from build123d import *

# Parameters (mm, degrees)
SKETCH1_W           = 31.86
SKETCH1_H           = 328
BOSS_EXTRUDE1_DEPTH = 5
SKETCH2_R           = 2.1
CUT_EXTRUDE1_DEPTH  = 10
CUT_EXTRUDE2_DEPTH  = 10
BOSS_EXTRUDE2_DEPTH = 5
SKETCH7_W           = 4.2
SKETCH7_H           = 5
SKETCH7_R           = 2.099999245
CUT_EXTRUDE3_DEPTH  = 5
SKETCH8_R           = 2.499996422
SKETCH8_R_2         = 2.499996502
SKETCH8_R_3         = 2.5
SKETCH8_W           = 40.200355047
SKETCH8_H           = 20
CUT_EXTRUDE4_DEPTH  = 10
CUT_EXTRUDE5_DEPTH  = 10
CUT_EXTRUDE6_DEPTH  = 10
SKETCH12_R          = 2.100000755
SKETCH12_R_2        = 2.1
SKETCH12_W          = 15.000005391
SKETCH12_H          = 5
SKETCH12_W_2        = 5
SKETCH12_H_2        = 40
CUT_EXTRUDE7_DEPTH  = 5
SKETCH15_W          = 40
SKETCH15_H          = 5
CUT_EXTRUDE8_DEPTH  = 5


with BuildPart() as part:
    # Sketch1 → Boss-Extrude1 (new body)
    with BuildSketch(Plane.XY):
        Rectangle(SKETCH1_W, SKETCH1_H)
    extrude(amount=BOSS_EXTRUDE1_DEPTH)

    # Sketch2 → Cut-Extrude1 (cut)
    with BuildSketch(Plane.XY.offset(5)):
        with Locations((0, 81.5)):
            Circle(SKETCH2_R)
    extrude(amount=-CUT_EXTRUDE1_DEPTH, mode=Mode.SUBTRACT)

    # Sketch3 → Cut-Extrude2 (cut)
    with BuildSketch(Plane.XY.offset(5)):
        Polygon((2.1, 164), (2.1, 159), (5, 159), (5, 149), (-5, 149), (-5, 159), (-2.1, 159), (-2.1, 164), align=None)
        Polygon((-2.1, -164), (-2.1, -159), (-5, -159), (-5, -149), (5, -149), (5, -159), (2.1, -159), (2.1, -164), align=None)
    extrude(amount=-CUT_EXTRUDE2_DEPTH, mode=Mode.SUBTRACT)

    # Sketch4 → Boss-Extrude2 (add)
    with BuildSketch(Plane(origin=(0, 0, 0), x_dir=(-1, 0, 0), z_dir=(0, 0, -1))):
        with BuildLine():
            Line((15.93, -164), (108.913444487, -164))
            Line((108.913444487, -164), (108.913444487, 109))
            Line((108.913444487, 109), (101.503490547, 109))
            ThreePointArc((101.503490547, 109), (62.423444487, 88.5), (23.343398428, 109))
            ThreePointArc((23.343398428, 109), (18.773737927, 117.266257257), (15.93, 126.273252357))
            Line((15.93, 126.273252357), (15.93, 109))
            Line((15.93, 109), (15.93, -164))
        make_face()
    extrude(amount=-BOSS_EXTRUDE2_DEPTH)

    # Sketch7 → Cut-Extrude3 (cut)
    with BuildSketch(Plane.XY.offset(5)):
        Polygon((-95.083444487, -159), (-90.883444487, -159), (-87.983444487, -159), (-87.983444487, -149), (-97.983444487, -149), (-97.983444487, -159), align=None)
        with Locations((-92.983444487, -161.5)):
            Rectangle(SKETCH7_W, SKETCH7_H)
        with Locations((0.021526005, 106.5)):
            Circle(SKETCH7_R)
    extrude(amount=-CUT_EXTRUDE3_DEPTH, mode=Mode.SUBTRACT)

    # Sketch8 → Cut-Extrude4 (cut)
    with BuildSketch(Plane.XY.offset(5)):
        with Locations((-38.679067758, 44.08)):
            Circle(SKETCH8_R)
        with Locations((-38.679067758, 33.92)):
            Circle(SKETCH8_R_2)
        with Locations((10.13, 44.08)):
            Circle(SKETCH8_R_3)
        with Locations((10.13, 33.92)):
            Circle(SKETCH8_R_3)
        with Locations((-14.269822477, 39)):
            Rectangle(SKETCH8_W, SKETCH8_H)
    extrude(amount=-CUT_EXTRUDE4_DEPTH, mode=Mode.SUBTRACT)

    # Sketch9 → Cut-Extrude5 (cut)
    with BuildSketch(Plane(origin=(0, 0, 0), x_dir=(-1, 0, 0), z_dir=(0, 0, -1))):
        with BuildLine():
            Line((4.37, 12), (4.37, 19))
            ThreePointArc((4.37, 19), (-15.63, 39), (4.37, 59))
            Line((4.37, 59), (4.37, 66))
            ThreePointArc((4.37, 66), (-22.63, 39), (4.37, 12))
        make_face()
    extrude(amount=-CUT_EXTRUDE5_DEPTH, mode=Mode.SUBTRACT)

    # Sketch10 → Cut-Extrude6 (cut)
    with BuildSketch(Plane(origin=(0, 0, 0), x_dir=(-1, 0, 0), z_dir=(0, 0, -1))):
        with BuildLine():
            Line((-15.93, 66), (-15.93, 56.801966184))
            ThreePointArc((-15.93, 56.801966184), (-6.773314432, 63.593221495), (4.37, 66))
            Line((4.37, 66), (4.25, 81.5))
            ThreePointArc((4.25, 81.5), (0, 77.25), (-4.25, 81.5))
            Line((-4.25, 81.5), (-15.93, 81.5))
            Line((-15.93, 81.5), (-15.93, 66))
        make_face()
    extrude(amount=-CUT_EXTRUDE6_DEPTH, mode=Mode.SUBTRACT)

    # Sketch12 → Cut-Extrude7 (cut)
    with BuildSketch(Plane(origin=(0, 0, 0), x_dir=(-1, 0, 0), z_dir=(0, 0, -1))):
        with Locations((30.403186809, -93.5)):
            Circle(SKETCH12_R)
        with Locations((79.236368236, -70)):
            Circle(SKETCH12_R_2)
        with Locations((54.236365541, -93.5)):
            Rectangle(SKETCH12_W, SKETCH12_H)
        with Locations((6.570008077, -93.5)):
            Rectangle(SKETCH12_W, SKETCH12_H)
        with Locations((79.236368236, -114)):
            Rectangle(SKETCH12_W_2, SKETCH12_H_2)
        with Locations((79.236368236, -26)):
            Rectangle(SKETCH12_W_2, SKETCH12_H_2)
    extrude(amount=-CUT_EXTRUDE7_DEPTH, mode=Mode.SUBTRACT)

    # Sketch15 → Cut-Extrude8 (cut)
    with BuildSketch(Plane.XY.offset(5)):
        with Locations((-61.674975637, 81.5)):
            Rectangle(SKETCH15_W, SKETCH15_H)
    extrude(amount=-CUT_EXTRUDE8_DEPTH, mode=Mode.SUBTRACT)


solid = part.part
The model under review builds one solid part; all positions refer to its coordinate system, in mm. Give positions to 0.01 mm unless a question says otherwise; leave off trailing zeros. Order: outer loops, then holes, each group sorted by start corner. A loop starts at its lowest first (then second) coordinate and runs counter-clockwise, first axis right, second up. Notation, with made-up numbers: M 48.25,-28 L 98.25,-28 A10 ccw 98.25,-15 Z; hole C -40,-36.5 d10. An arc over 180 degrees is marked long. Answer in a Markdown table with one row per item. Add a question column.
1. Add section B-B on z = 0.8. Count the separate pieces of the cut face and the enclosed holes in it, plus the area to 3 significant figures.
2. Mouldability with a two-part tool opening along Y and no side actions: class faces 1 (the cylindrical face through (6.92, 14.474, 2.465)), 2 (the flat face through (-46, -34, 0)) as released by +Y, released by -Y, zero draft, split by the parting line, or undercut.
3. To check wall thickness, follow line 1 along Y through (x, z) = (-11.5, 4.7); line 2 along Y through (x, z) = (-63, 4.65); line 3 along X through (y, z) = (-130, 1.45). State the ranges of each line that lie inside material, in increasing order.
4. Add section A-A on y = -21. State the section outline as (x, z) points, plus the area to 3 significant figures.
5. For pin 1 Ø2 at (x, z) = (-21, 2.5) entering from +Y; pin 2 Ø1.5 at (x, z) = (-97, 1.5) entering from +Y; pin 3 Ø6 at (x, y) = (-74.5, 49) entering from -Z; pin 4 Ø1.5 at (y, z) = (162.5, 3) entering from -X, all flat-tipped, find the tip position at first contact; note any pin that passes through.
The answers:
| question | item | result |
|---|---|---|
| 1 | separate pieces | 1 |
| 1 | enclosed holes | 14 |
| 1 | area | 32,000 mm2 |
| 2 | face 1 | undercut |
| 2 | face 2 | zero draft |
| 3 | line 1 | -164 to -96, -91 to 29, 49 to 164 |
| 3 | line 2 | -164 to 79, 84 to 88.5 |
| 3 | line 3 | -108.91 to -81.74, -76.74 to 15.93 |
| 4 | outline | M -108.91,0 L -81.74,0 L -81.74,5 L -108.91,5 Z; M -76.74,0 L 15.93,0 L 15.93,5 L -76.74,5 Z |
| 4 | area | 599 mm2 |
| 5 | pin 1 | y = 114.63 |
| 5 | pin 2 | y = 104.25 |
| 5 | pin 3 | z = 0 |
| 5 | pin 4 | x = -15.93 |
